Could you check a few things on this model? Use its own coordinates, in mm. A direction names the side the tool comes from. Coordinates: 2 decimals unless noted, no trailing zeros. Loops run counter-clockwise (first coordinate to the right, second up) from the corner with the lowest first, then second, coordinate; pieces in that order, holes last. Notation, with made-up numbers: M -10.5,27.25 L 38.5,27.25 A29 ccw 38.5,53.25 Z; hole C 2,71 d1. An arc over 180 degrees is marked long. Use one line per item in the form item = value. Start each with the question number.
```python
from build123d import *

# Parameters (mm, degrees)
SKETCH_3_W               = 36
SKETCH_3_H               = 42
SKETCH_3_W_2             = 16
SKETCH_3_H_2             = 22
CUT_EXTRUDE_1_DEPTH      = 21
SKETCH_4_W               = 16
SKETCH_4_H               = 4
CUT_EXTRUDE_2_DEPTH      = 27
CUT_EXTRUDE_2_DEPTH_BACK = 27


with BuildPart() as part:
    # Sketch 1 → Revolve 1 (revolve)
    with BuildSketch(Plane.XY, mode=Mode.PRIVATE) as revolve_1_sk:
        with BuildLine():
            Line((0, 0), (0, 10.08))
            Line((0, 10.08), (0.92, 11))
            Line((0.92, 11), (12, 11))
            Line((12, 11), (12, 13.1))
            ThreePointArc((12, 13.1), (12.117157288, 13.382842712), (12.4, 13.5))
            Line((12.4, 13.5), (27.6, 13.5))
            ThreePointArc((27.6, 13.5), (27.882842712, 13.382842712), (28, 13.1))
            Line((28, 13.1), (28, 10.7))
            Line((28, 10.7), (29, 10.7))
            Line((29, 10.7), (29, 10.2))
            Line((29, 10.2), (29.3, 10.7))
            Line((29.3, 10.7), (470.7, 10.7))
            Line((470.7, 10.7), (471, 10.2))
            Line((471, 10.2), (471, 10.7))
            Line((471, 10.7), (472, 10.7))
            Line((472, 10.7), (472, 13.1))
            ThreePointArc((472, 13.1), (472.117157288, 13.382842712), (472.4, 13.5))
            Line((472.4, 13.5), (487.6, 13.5))
            ThreePointArc((487.6, 13.5), (487.882842712, 13.382842712), (488, 13.1))
            Line((488, 13.1), (488, 0))
            Line((488, 0), (0, 0))
        make_face()
    revolve(revolve_1_sk.sketch.rotate(Axis((488, 0, 0), (-1, 0, 0)), 270), axis=Axis((488, 0, 0), (-1, 0, 0)))

    # Sketch 2 → Revolve 2 (revolve)
    with BuildSketch(Plane.XY, mode=Mode.PRIVATE) as revolve_2_sk:
        Polygon((488, 0), (488, 10.85), (490, 10.85), (490, 11), (508, 11), (509, 10), (509, 0), align=None)
    revolve(revolve_2_sk.sketch.rotate(Axis((509, 0, 0), (-1, 0, 0)), 270), axis=Axis((509, 0, 0), (-1, 0, 0)))

    # Sketch 3 → Cut-Extrude 1 (cut)
    with BuildSketch(Plane(origin=(509, 0, 0), x_dir=(0, 0, -1), z_dir=(1, 0, 0))):
        Rectangle(SKETCH_3_W, SKETCH_3_H)
        Rectangle(SKETCH_3_W_2, SKETCH_3_H_2, mode=Mode.SUBTRACT)
    extrude(amount=-CUT_EXTRUDE_1_DEPTH, mode=Mode.SUBTRACT)

    # Sketch 4 → Cut-Revolve 1 (revolve, cut)
    with BuildSketch(Plane(origin=(500, 0, 0), x_dir=(0, 0, -1), z_dir=(1, 0, 0)), mode=Mode.PRIVATE) as cut_revolve_1_sk:
        with Locations((0, 2)):
            Rectangle(SKETCH_4_W, SKETCH_4_H)
    revolve(cut_revolve_1_sk.sketch.rotate(Axis((500, 0, -8), (0, 0, 1)), 270), axis=Axis((500, 0, -8), (0, 0, 1)), mode=Mode.SUBTRACT)

    # Sketch 5 → Cut-Revolve 2 (revolve, cut)
    with BuildSketch(Plane.XY, mode=Mode.PRIVATE) as cut_revolve_2_sk:
        Polygon((20, 13.5), (24.864, 13.5), (24.283, 12.919), (24.283, 5.5), (20, 5.5), align=None)
    revolve(cut_revolve_2_sk.sketch.rotate(Axis((20, 5.5, 0), (0, 1, 0)), 270), axis=Axis((20, 5.5, 0), (0, 1, 0)), mode=Mode.SUBTRACT)

    # Sketch 6 → Cut-Revolve 3 (revolve, cut)
    with BuildSketch(Plane.XY, mode=Mode.PRIVATE) as cut_revolve_3_sk:
        Polygon((480, 13.5), (484.864, 13.5), (484.283, 12.919), (484.283, 5.5), (480, 5.5), align=None)
    revolve(cut_revolve_3_sk.sketch.rotate(Axis((480, 5.5, 0), (0, 1, 0)), 270), axis=Axis((480, 5.5, 0), (0, 1, 0)), mode=Mode.SUBTRACT)

    # Sketch 7 → Cut-Extrude 2 (cut, two sides: drawn at the far end of the back side and taken through both)
    with BuildSketch(Plane(origin=(0, 0, 0), x_dir=(1, 0, 0), z_dir=(0, 1, 0)).offset(-CUT_EXTRUDE_2_DEPTH_BACK)):
        Polygon((-4, -13.5), (21.5, -13.5), (20.5, -12.5), (-2, -12.5), (-2, 12.5), (20.5, 12.5), (21.5, 13.5), (-4, 13.5), align=None)
    extrude(amount=CUT_EXTRUDE_2_DEPTH + CUT_EXTRUDE_2_DEPTH_BACK, mode=Mode.SUBTRACT)

    # Sketch 8 → Cut-Revolve 4 (revolve, cut)
    with BuildSketch(Plane.XY, mode=Mode.PRIVATE) as cut_revolve_4_sk:
        Polygon((0, 0), (0, 4), (39, 4), (39, 10), (461, 10), (461, 0), align=None)
    revolve(cut_revolve_4_sk.sketch.rotate(Axis((461, 0, 0), (-1, 0, 0)), 270), axis=Axis((461, 0, 0), (-1, 0, 0)), mode=Mode.SUBTRACT)


solid = part.part
```
Item 1: I'm going to push flat-ended pins straight in: P1, Ø2.5, axis at x = 21, z = 1, coming from the +Y side; P2, Ø8, axis at x = 218.5, z = -0.5, coming from the -Y side; P3, Ø7, axis at y = 0, z = 0, coming from the -X side. Where does each tip first touch, or does it pass through?
Item 2: Please list where these lines run through material, in increasing order: line 1 along X through (y, z) = (7.5, 0); line 2 along Y through (x, z) = (235.5, 0); line 3 along X through (y, z) = (-12, 2.5).
Item 3: I want a section at A-A (x = 312). Write out the boundary of the cut face in (y, z), plus the area to 3 significant figures.
Item 4: Thinking about a two-plate mould opening in Y: for faces 1 (the cylindrical face through (28.507, -10.446, -2.32)), 2 (the cylindrical face through (496, 0, 0)), 3 (the flat face through (496, 2, -8)), which applies, pulls with the +Y half, pulls with the -Y half, needs draft (parallel to the pull), parting line crosses it, or undercut?
Item 5: For faces 4 (the flat face through (16, 0, 12.5)), 5 (the cylindrical face through (499, 11, 0)), 6 (the cylindrical face through (19.773, -3.905, -0.867)), 7 (the flat face through (472, 0, 11)), 8 (the cylindrical face through (499, -11, 0)), which set-ups out of +Z, -Z, +X, -X, +Y, -Y let a thin tool reach every point of the face, with its end or its side?
Worked answers:
q1.P1 = 5.5
q1.P2 = -10.7
q1.P3 = 461
q2.line_1 = 0 to 15.72, 24.28 to 39, 461 to 475.72, 484.28 to 509
q2.line_2 = -10.7 to -10, 10 to 10.7
q2.line_3 = 12 to 28, 472 to 488
q3.outline = C 0,0 d21.4; hole C 0,0 d20
q3.area = 45.5 mm²
q4.face_1 = parting line crosses it
q4.face_2 = undercut
q4.face_3 = needs draft
q5.face_4 = +Z, -X, +Y, -Y
q5.face_5 = +X, +Y
q5.face_6 = -X
q5.face_7 = none
q5.face_8 = +X, -Y
